```python
from build123d import *

# Parameters (mm, degrees)
F0_W     = 25.4
F0_H     = 6.35
F0_R     = 1.5875
F1_DEPTH = 12.7
F2_W     = 3.784558
F2_H     = 3.142819
F3_DEPTH = 25.4
F4_W     = 5.247167
F4_H     = 3.388975
F5_DEPTH = 25.4
F6_R     = 2.113267
F7_DEPTH = 25.4


with BuildPart() as f1:
    # F0 (on Front) → F1 (new body)
    with BuildSketch(Plane.XZ):
        with Locations((4.764033, 0)):
            Rectangle(F0_W, F0_H)
        with Locations((-1.585967, 0)):
            Circle(F0_R, mode=Mode.SUBTRACT)
        with Locations((11.114033, 0)):
            Circle(F0_R, mode=Mode.SUBTRACT)
    extrude(amount=F1_DEPTH)

    # F2 (on face) → F3 (cut)
    with BuildSketch(Plane(origin=(0, 0, -3.175), x_dir=(1, 0, 0), z_dir=(0, 0, -1))):
        with Locations((6.177249, 5.877707)):
            Rectangle(F2_W, F2_H)
    extrude(amount=-F3_DEPTH, mode=Mode.SUBTRACT)

    # F4 (on face) → F5 (cut)
    with BuildSketch(Plane(origin=(-7.935967, 0, 0), x_dir=(0, -1, 0), z_dir=(-1, 0, 0))):
        with Locations((6.250942, -0.213469)):
            Rectangle(F4_W, F4_H)
    extrude(amount=-F5_DEPTH, mode=Mode.SUBTRACT)

    # F6 (on face) → F7 (cut)
    with BuildSketch(Plane.XZ):
        with Locations((5.720744, 0)):
            Circle(F6_R)
    extrude(amount=-F7_DEPTH, mode=Mode.SUBTRACT)


solid = f1.part
```
Can you work these out from the model? Positions are in its coordinate system, mm. A direction names the side the tool comes from. Give positions to 0.01 mm unless a question says otherwise; leave off trailing zeros. Loops run counter-clockwise (first coordinate to the right, second up) from the corner with the lowest first, then second, coordinate; pieces in that order, holes last. Notation, with made-up numbers: M 37.5,-27 L 71.5,-27 A25 cw 71.5,2 Z; hole C 18.5,31.25 d6. An arc over 180 degrees is marked long. Answer in a Markdown table with one row per item.
1. Suppose I cut it at B-B on x = 4.75. Write out the boundary of the cut face in (y, z) (3 decimals).
Taken from the geometry:
| item | result |
|---|---|
| outline | M -12.7,-3.175 L -7.449,-3.175 L -7.449,-1.908 L -8.875,-1.908 L -8.875,1.481 L -7.449,1.481 L -7.449,3.175 L -12.7,3.175 Z; M -4.306,-3.175 L 0,-3.175 L 0,3.175 L -4.306,3.175 L -4.306,1.481 L -3.627,1.481 L -3.627,-1.908 L -4.306,-1.908 Z |
2. Suppose I cut it at D-D on y = -9.75. Write out the boundary of the cut face in (x, z) (1 decimal), plus the area to 3 significant figures.
Taken from the geometry:
| item | result |
|---|---|
| outline | M -7.9,-3.2 L 17.5,-3.2 L 17.5,3.2 L -7.9,3.2 Z; hole C -1.6,0 d3.2; hole C 11.1,0 d3.2 |
| area | 145 mm² |
3. Suppose I cut it at A-A on z = 0. Write out the boundary of the cut face in (x, y).
Taken from the geometry:
| item | result |
|---|---|
| outline | M -7.94,-12.7 L -3.17,-12.7 L -3.17,-8.87 L -7.94,-8.87 Z; M -7.94,-3.63 L -3.17,-3.63 L -3.17,0 L -7.94,0 Z; M 0,-12.7 L 9.53,-12.7 L 9.53,-8.87 L 0,-8.87 Z; M 0,-3.63 L 9.53,-3.63 L 9.53,0 L 0,0 Z; M 12.7,-12.7 L 17.46,-12.7 L 17.46,-8.87 L 12.7,-8.87 Z; M 12.7,-3.63 L 17.46,-3.63 L 17.46,0 L 12.7,0 Z |
4. Thinking about a two-plate mould opening in Y: for faces 4 (the flat face through (5, 0, 0)), 5 (the flat face through (5, -8, -3.175)), 6 (the flat face through (-5, -6, 1.481)), which applies, released by +Y, released by -Y, zero draft, split by the parting line, or undercut?
Taken from the geometry:
| item | result |
|---|---|
| face 4 | released by +Y |
| face 5 | zero draft |
| face 6 | undercut |
5. For pin 1 Ø2.5 at (x, z) = (-1.5, 0) entering from +Y, with a flat end and sliding along its axis, tell me the tip position at first contact or that it passes through.
Taken from the geometry:
| item | result |
|---|---|
| pin 1 | passes through |
6. Suppose I cut it at C-C on x = 13.5. Write out the boundary of the cut face in (y, z) (3 decimals), plus the area to 3 significant figures.
Taken from the geometry:
| item | result |
|---|---|
| outline | M -12.7,-3.175 L 0,-3.175 L 0,3.175 L -12.7,3.175 Z; hole M -8.875,-1.908 L -3.627,-1.908 L -3.627,1.481 L -8.875,1.481 Z |
| area | 62.9 mm² |
7. If I drill on line 1 along X through (y, z) = (-9.75, 0); line 2 along Y through (x, z) = (5.5, -2.75); line 3 along Z through (x, y) = (-4.25, -7) (3 decimals), over which ranges is the centre line in solid material (lowest first)?
Taken from the geometry:
| item | result |
|---|---|
| line 1 | x = -7.94 to -3.17, 0 to 9.53, 12.7 to 17.46 |
| line 2 | y = -12.7 to -7.45, -4.31 to 0 |
| line 3 | z = -3.175 to -1.908, 1.481 to 3.175 |
8. Which directions (+Z, -Z, +X, -X, +Y, -Y) give clear straight access to the entire face, cutting with the end or side of a thin tool? Please do faces 1 (the flat face through (5, -12.7, 0)), 2 (the flat face through (6, -7.449, -3)), 3 (the flat face through (5, -8, -1.908)).
Taken from the geometry:
| item | result |
|---|---|
| face 1 | +Z, -Z, +X, -X, -Y |
| face 2 | +Z, -Z |
| face 3 | +X, -X |
